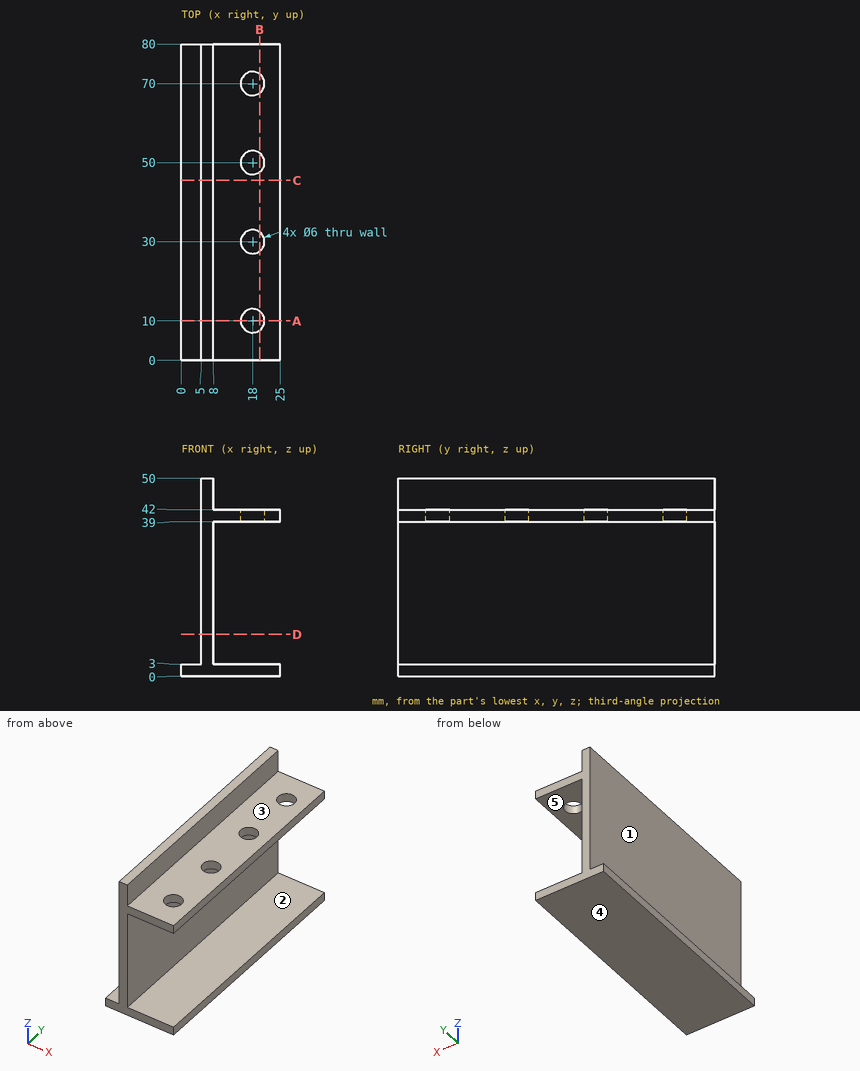
Verification items for this drawing (mm, ordinates from the low corner). A direction names the side the tool comes from. Round coordinates to 2 decimals unless told otherwise and drop trailing zeros. Loops run counter-clockwise (first coordinate to the right, second up) from the corner with the lowest first, then second, coordinate; pieces in that order, holes last. Notation, with made-up numbers: (76.5, 64) - (126.5, 64) arc R19 ccw to (126.5, 93) - close; hole circle Ø7 at (88.25, 58.25). An arc over 180 degrees is marked (long way). Answer as CSV lines item,"result". Start each with the question number.
Item 1: Set-up check for the marked faces 4 and 5: record each of +Z, -Z, +X, -X, +Y, -Y from which the full face is reachable in a straight line by a thin tool's end or side.
Item 2: Section check C-C (y = 45.5). Record the boundary of the cut face in (x, z), and give its area (3 significant figures).
Item 3: Scan lines: line 1 (Y direction, x = 18, z = 40.8); line 2 (Z direction, x = 13.75, y = 39); line 3 (Z direction, x = 4, y = 26). Record each from-to range of solid material in increasing order. Write a range as [from, to].
Item 4: Section check A-A (y = 10). Record the boundary of the cut face in (x, z), and give its area (3 significant figures).
Item 5: Release check for a two-part mould opening along Z. For the marked faces 1, 2 and 3 record: +Z half, -Z half, draft (parallel to the pull), parting line (faces both ways), or undercut.
Item 6: Depth check by flat-ended pin: P1, Ø10, axis at y = 27.5, z = 18.5, coming from the +X side; P2, Ø1.5, axis at x = 2.5, y = 55.5, coming from the +Z side; P3, Ø13.5, axis at x = 18.5, y = 40, coming from the +Z side; P4, Ø6, axis at x = 13.5, z = 23.5, coming from the -Y side. Enter the tip coordinate at first touch or a pass-through.
Item 7: Section check B-B (x = 19.75). Record the boundary of the cut face in (y, z).
Item 8: Section check D-D (z = 10.5). Record the boundary of the cut face in (x, y), and give its area (3 significant figures).
Report:
1,face 4,"-Z, +X, -X, +Y, -Y"
1,face 5,"+X, +Y, -Y"
2,outline,"(0, 0) - (25, 0) - (25, 3) - (8, 3) - (8, 39) - (25, 39) - (25, 42) - (8, 42) - (8, 50) - (5, 50) - (5, 3) - (0, 3) - close"
2,area,"267 mm2"
3,line 1,"y = [0, 7], [13, 27], [33, 47], [53, 67], [73, 80]"
3,line 2,"z = [0, 3], [39, 42]"
3,line 3,"z = [0, 3]"
4,outline,"(0, 0) - (25, 0) - (25, 3) - (8, 3) - (8, 39) - (15, 39) - (15, 42) - (8, 42) - (8, 50) - (5, 50) - (5, 3) - (0, 3) - close; (21, 39) - (25, 39) - (25, 42) - (21, 42) - close"
4,area,"249 mm2"
5,face 1,"draft"
5,face 2,"undercut"
5,face 3,"+Z half"
6,P1,"stops at x = 8"
6,P2,"stops at z = 3"
6,P3,"stops at z = 42"
6,P4,"passes through"
7,outline,"(0, 0) - (80, 0) - (80, 3) - (0, 3) - close; (0, 39) - (7.56, 39) - (7.56, 42) - (0, 42) - close; (12.44, 39) - (27.56, 39) - (27.56, 42) - (12.44, 42) - close; (32.44, 39) - (47.56, 39) - (47.56, 42) - (32.44, 42) - close; (52.44, 39) - (67.56, 39) - (67.56, 42) - (52.44, 42) - close; (72.44, 39) - (80, 39) - (80, 42) - (72.44, 42) - close"
8,outline,"(5, 0) - (8, 0) - (8, 80) - (5, 80) - close"
8,area,"240 mm2"
